The listing builds one solid part. Answer for the finished solid, in the listing's coordinates (mm). Give positions to 0.01 mm unless a question says otherwise; leave off trailing zeros. Order: outer loops, then holes, each group sorted by start corner. A loop starts at its lowest first (then second) coordinate and runs counter-clockwise, first axis right, second up. Notation, with made-up numbers: (78.25, -12) -> (119.25, -12) arc R24 ccw to (119.25, 6) -> close; hole circle Ø10 at (65.5, 48.5). An arc over 180 degrees is marked (long way). Answer as a JSON object with one key per item and string values. Group by question number.
```python
from build123d import *

# Parameters (mm, degrees)
F1_DEPTH      = 2
F2_DEPTH      = 5
F2_DEPTH_BACK = 2
F3_DEPTH      = 5


with BuildPart() as f1:
    # F0 (on Front) → F1 (new body)
    with BuildSketch(Plane.XZ):
        with BuildLine():
            Line((4, 0), (5, 0))
            ThreePointArc((5, 0), (3.9667667015, 3.043807145), (1.2940952255, 4.8296291314))
            Line((1.2940952255, 4.8296291314), (1.0352761804, 3.8637033052))
            ThreePointArc((1.0352761804, 3.8637033052), (3.1734133612, 2.435045716), (4, 0))
        make_face()
        with BuildLine():
            Line((1.0352761804, 3.8637033052), (1.2940952255, 4.8296291314))
            ThreePointArc((1.2940952255, 4.8296291314), (1.0821980697, 4.8814800356), (0.8682408883, 4.9240387651))
            Line((0.8682408883, 4.9240387651), (0.6945927107, 3.939231012))
            ThreePointArc((0.6945927107, 3.939231012), (0.8657584558, 3.9051840285), (1.0352761804, 3.8637033052))
        make_face()
        with BuildLine():
            Line((0.6945927107, 3.939231012), (0.8682408883, 4.9240387651))
            ThreePointArc((0.8682408883, 4.9240387651), (0, 5), (-0.8682408883, 4.9240387651))
            Line((-0.8682408883, 4.9240387651), (-0.6945927107, 3.939231012))
            ThreePointArc((-0.6945927107, 3.939231012), (0, 4), (0.6945927107, 3.939231012))
        make_face()
        with BuildLine():
            ThreePointArc((-0.8682408883, 4.9240387651), (-1.0821980697, 4.8814800356), (-1.2940952255, 4.8296291314))
            Line((-1.2940952255, 4.8296291314), (-1.0352761804, 3.8637033052))
            ThreePointArc((-1.0352761804, 3.8637033052), (-0.8657584558, 3.9051840285), (-0.6945927107, 3.939231012))
            Line((-0.6945927107, 3.939231012), (-0.8682408883, 4.9240387651))
        make_face()
        with BuildLine():
            ThreePointArc((-1.2940952255, 4.8296291314), (-3.9667667015, 3.043807145), (-5, 0))
            Line((-5, 0), (-4, 0))
            ThreePointArc((-4, 0), (-3.1734133612, 2.435045716), (-1.0352761804, 3.8637033052))
            Line((-1.0352761804, 3.8637033052), (-1.2940952255, 4.8296291314))
        make_face()
    extrude(amount=-F1_DEPTH)

    # F0 (on Front) → F2 (join, two sides)
    with BuildSketch(Plane.XZ) as f2_sk:
        with BuildLine():
            Line((0.6945927107, 3.939231012), (0.8682408883, 4.9240387651))
            ThreePointArc((0.8682408883, 4.9240387651), (0, 5), (-0.8682408883, 4.9240387651))
            Line((-0.8682408883, 4.9240387651), (-0.6945927107, 3.939231012))
            ThreePointArc((-0.6945927107, 3.939231012), (0, 4), (0.6945927107, 3.939231012))
        make_face()
        with BuildLine():
            ThreePointArc((-0.8682408883, 4.9240387651), (0, 5), (0.8682408883, 4.9240387651))
            Line((0.8682408883, 4.9240387651), (0.9550649772, 5.4164426416))
            ThreePointArc((0.9550649772, 5.4164426416), (0, 5.5), (-0.9550649772, 5.4164426416))
            Line((-0.9550649772, 5.4164426416), (-0.8682408883, 4.9240387651))
        make_face()
    extrude(amount=F2_DEPTH)
    extrude(f2_sk.sketch, amount=-F2_DEPTH_BACK)

    # F0 (on Front) → F3 (join)
    with BuildSketch(Plane.XZ):
        with BuildLine():
            Line((4, 0), (5, 0))
            ThreePointArc((5, 0), (3.9667667015, 3.043807145), (1.2940952255, 4.8296291314))
            Line((1.2940952255, 4.8296291314), (1.0352761804, 3.8637033052))
            ThreePointArc((1.0352761804, 3.8637033052), (3.1734133612, 2.435045716), (4, 0))
        make_face()
        with BuildLine():
            ThreePointArc((-1.2940952255, 4.8296291314), (-3.9667667015, 3.043807145), (-5, 0))
            Line((-5, 0), (-4, 0))
            ThreePointArc((-4, 0), (-3.1734133612, 2.435045716), (-1.0352761804, 3.8637033052))
            Line((-1.0352761804, 3.8637033052), (-1.2940952255, 4.8296291314))
        make_face()
    extrude(amount=F3_DEPTH)

    # F5 (on offset) → F6 (revolve)
    with BuildSketch(Plane.XZ.offset(3)):
        with BuildLine():
            Line((0, 6), (0, 5))
            ThreePointArc((0, 5), (0.3535533906, 5.1464466094), (0.5, 5.5))
            ThreePointArc((0.5, 5.5), (0.3535533906, 5.8535533906), (0, 6))
        make_face()
    revolve(axis=Axis((0, -3, 4.2273908738), (0, 0, 1)))


solid = f1.part
```
(1) A cutting plane is placed at A-A (y = -4). Determine the outline of the cut face in (x, z), and give its area (3 significant figures).
(2) A cutting plane is placed at C-C (y = 1.5). Determine the outline of the cut face in (x, z), and give its area (3 significant figures).
(3) Find the intervals of material crossed by line 1 along X through (y, z) = (0, 3.65); line 2 along X through (y, z) = (-3, 1.55); line 3 along Z through (x, y) = (-2.25, 0.5), in increasing order. Write a range as [from, to].
(4) A cutting plane is placed at D-D (z = 2.25). Determine the outline of the cut face in (x, y).
(5) A cutting plane is placed at B-B (z = 1.65). Determine the outline of the cut face in (x, y).
(6) For a pull along X with two mould halves and no side action, classify faces 1 (the flat face through (1.166, -2.465, 4.353)), 2 (the cylindrical face through (0, -1.5, 5.5)), 3 (the flat face through (0, -5, 5)), 4 (the flat face through (-1.163, -2.465, 4.34)) as +X half, -X half, draft (parallel to the pull), parting line (faces both ways), or undercut.
(7) Flat-ended cylindrical pins translate along their axes: pin 1 Ø4 at (x, y) = (-0.5, 1) entering from -Z; pin 2 Ø2 at (y, z) = (-1.5, 2.5) entering from +X. Find the tip coordinate at first contact, or state that the pin passes through.
Check sheet entries:
{
 "1": {"outline": "(-5, 0) -> (-4, 0) arc R4 cw to (-1.04, 3.86) -> (-1.29, 4.83) arc R5 ccw to start; (-0.96, 5.42) -> (-0.69, 3.94) arc R4 cw to (0.69, 3.94) -> (0.96, 5.42) arc R5.5 ccw to start; (1.04, 3.86) arc R4 cw to (4, 0) -> (5, 0) arc R5 ccw to (1.29, 4.83) -> close", "area": "14.3 mm2"},
 "2": {"outline": "(-5, 0) -> (-4, 0) arc R4 cw to (4, 0) -> (5, 0) arc R5 ccw to (0.87, 4.92) -> (0.96, 5.42) arc R5.5 ccw to (-0.96, 5.42) -> (-0.87, 4.92) arc R5 ccw to start", "area": "15.1 mm2"},
 "3": {"line 1": "x = [-3.42, -1.64], [1.64, 3.42]", "line 2": "x = [-4.75, -3.69], [3.69, 4.75]", "line 3": "z = [3.31, 4.47]"},
 "4": {"outline": "(-4.47, -5) -> (-3.31, -5) -> (-3.31, 2) -> (-4.47, 2) -> close; (3.31, -5) -> (4.47, -5) -> (4.47, 2) -> (3.31, 2) -> close"},
 "5": {"outline": "(-4.72, -5) -> (-3.64, -5) -> (-3.64, 2) -> (-4.72, 2) -> close; (3.64, -5) -> (4.72, -5) -> (4.72, 2) -> (3.64, 2) -> close"},
 "6": {"face 1": "undercut", "face 2": "parting line", "face 3": "draft", "face 4": "undercut"},
 "7": {"pin 1": "stops at z = 3.12", "pin 2": "stops at x = 4.77"}
}
